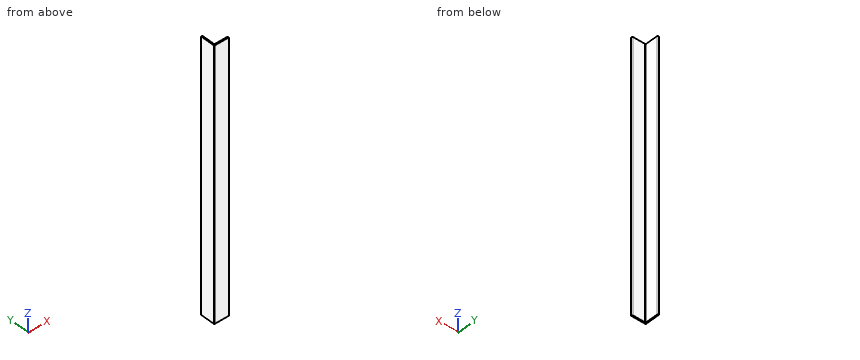
```python
from build123d import *

# Parameters (mm, degrees)
BOSS_EXTRUDE1_DEPTH = 350
FILLET1_R           = 1
FILLET2_R           = 0.5


with BuildPart() as part:
    # Sketch1 → Boss-Extrude1 (new body)
    with BuildSketch(Plane.XY):
        Polygon((0, 0), (0, 19.05), (1.5875, 19.05), (1.5875, 1.5875), (19.05, 1.5875), (19.05, 0), align=None)
    extrude(amount=BOSS_EXTRUDE1_DEPTH)

    # Fillet1
    fillet1_edges = [part.edges().sort_by_distance(p)[0] for p in [
        (1.5875, 19.05, 175),
        (1.5875, 1.5875, 175),
        (19.05, 1.5875, 175),
    ]]
    fillet(fillet1_edges, radius=FILLET1_R)

    # Fillet2
    fillet2_edges = [part.edges().sort_by_distance(p)[0] for p in [
        (0, 0, 175),
    ]]
    fillet(fillet2_edges, radius=FILLET2_R)


solid = part.part
```
CAD build for the part. Positions are in the model's coordinates, mm. Round coordinates to 2 decimals unless told otherwise and drop trailing zeros. Write each loop counter-clockwise with the first axis right and the second up, starting at its lowest first coordinate (ties: lowest second). Pieces come first, ordered by that corner, then holes. Notation, with made-up numbers: (-18, 33) - (24, 33) arc R23 ccw to (24, 55) - close; hole circle Ø5 at (-11.75, -19.75). An arc over 180 degrees is marked (long way). Write item = value, one per line. Start each with the question number.
Q1. Probe L1, parallel to X at y = 3.75, z = 54.5; L2, parallel to X at y = 2, z = 116.5. List the from-to ranges inside material, lowest first. Write a range as from..to.
Q2. Band-saw the part on B-B (x = 10.25). Give the cut face in (y, z), then the cut area to 3 significant figures.
Q3. Band-saw the part on A-A (z = 225). Give the cut face in (x, y).
Q4. Drop flat-ended pins along their axis: pin 1 (1 mm diameter, centred on y = 11, z = 296, fed in from +X); pin 2 (7.5 mm diameter, centred on x = 6.5, z = 178, fed in from +Y). Give the stop position or say it passes through.
Answers below:
q1.L1 = 0..1.59
q1.L2 = 0..1.78
q2.outline = (0, 0) - (1.59, 0) - (1.59, 350) - (0, 350) - close
q2.area = 556 mm2
q3.outline = (0, 0.5) arc R0.5 ccw to (0.5, 0) - (19.05, 0) - (19.05, 0.59) arc R1 ccw to (18.05, 1.59) - (2.59, 1.59) arc R1 cw to (1.59, 2.59) - (1.59, 18.05) arc R1 ccw to (0.59, 19.05) - (0, 19.05) - close
q4.pin_1 = 1.59
q4.pin_2 = 1.59
